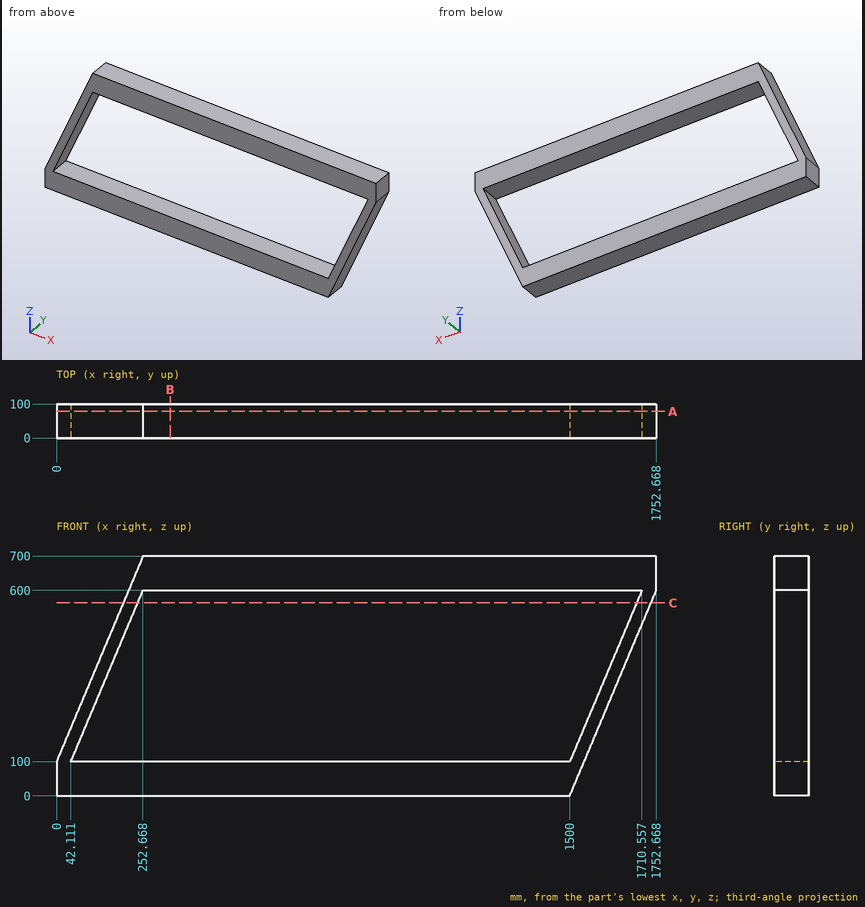
For this review, use the dimensioned drawing (mm, ordinates from the lowest corner) and the shaded views. Coordinates: 2 decimals unless noted, no trailing zeros. Order: outer loops, then holes, each group sorted by start corner. A loop starts at its lowest first (then second) coordinate and runs counter-clockwise, first axis right, second up. Notation, with made-up numbers: (14.5, -18.75) - (51.5, -18.75) arc R18 ccw to (51.5, -0.75) - close; hole circle Ø6 at (30, 89). An arc over 180 degrees is marked (long way). Answer as a JSON object with one key per item and string values. Group by question number.
1. We need section A-A on y = 78.5. State the section outline as (x, z) points.
2. We need section C-C on z = 563.5. State the section outline as (x, y) points, then the cut area to 3 significant figures.
3. We need section B-B on x = 332. State the section outline as (y, z) points, then the cut area to 3 significant figures.
4. Clearance check with flat-ended pins moving along their axes: P1, Ø8, axis at y = 44, z = 537.5, coming from the -X side; P2, Ø1.5, axis at x = 176, y = 29, coming from the +Z side; P3, Ø10, axis at y = 81, z = 602.5, coming from the -X side (1 decimal). State where each tip first meets the part, or that it passes through.
5. For probe 1 along Z at (x, y) = (1483.5, 37); probe 2 along Z at (x, y) = (101, 83); probe 3 along X at (y, z) = (32.5, 353), list the stretches that pass through material, from the lowest coordinate up.
Final values:
{
 "1": {"outline": "(0, 0) - (1500, 0) - (1752.67, 600) - (1752.67, 700) - (252.67, 700) - (0, 100) - close; hole (42.11, 100) - (1500, 100) - (1710.56, 600) - (252.67, 600) - close"},
 "2": {"outline": "(195.19, 0) - (237.3, 0) - (237.3, 100) - (195.19, 100) - close; (1695.19, 0) - (1737.3, 0) - (1737.3, 100) - (1695.19, 100) - close", "area": "8,420 mm²"},
 "3": {"outline": "(0, 0) - (100, 0) - (100, 100) - (0, 100) - close; (0, 600) - (100, 600) - (100, 700) - (0, 700) - close", "area": "20,000 mm²"},
 "4": {"P1": "x = 182.55", "P2": "z = 519.72", "P3": "x = 209.5"},
 "5": {"probe 1": "0 to 100, 600 to 700", "probe 2": "0 to 100, 239.84 to 339.84", "probe 3": "106.54 to 148.65, 1606.54 to 1648.65"}
}
